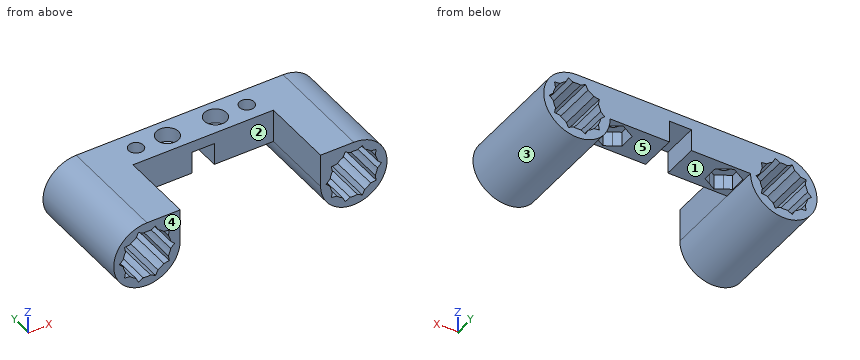
from build123d import *

# Parameters (mm, degrees)
F0_R            = 6.5
F1_DEPTH        = 25
F2_W            = 19
F2_H            = 9
F3_DEPTH        = 15
F4_R            = 2
F5_DEPTH        = 18.001
F7_DEPTH        = 25.001
F7_COPIES_COUNT = 10
F9_DEPTH        = 4
F10_DEPTH       = 5
F12_D           = 6
F12_DEPTH       = 4
F12_TIP         = 1.8025818571
F13_W           = 3
F13_H           = 6
F14_DEPTH       = 30.001


# Not quite as in the source:
# - a pattern or mirror of a feature is missing from the dataset's text; its kind, count and spacing are read off the source's solid


with BuildPart() as f1:
    # F0 (on Front) → F1 (new body)
    with BuildSketch(Plane.XZ):
        with BuildLine():
            Line((-19, 0), (0, 0))
            Line((0, 0), (0, 9))
            Line((0, 9), (-28, 9))
            ThreePointArc((-28, 9), (-21.6360389693, 6.3639610307), (-19, 0))
        make_face()
        with BuildLine():
            ThreePointArc((-28, 9), (-34.3639610307, -6.3639610307), (-19, 0))
            ThreePointArc((-19, 0), (-21.6360389693, 6.3639610307), (-28, 9))
        make_face()
        with Locations((-28, 0)):
            Circle(F0_R, mode=Mode.SUBTRACT)
    extrude(amount=F1_DEPTH)

    # F2 (on face) → F3 (cut)
    with BuildSketch(Plane.XZ.offset(25)):
        with Locations((-9.5, 4.5)):
            Rectangle(F2_W, F2_H)
    extrude(amount=-F3_DEPTH, mode=Mode.SUBTRACT)

    # F4 (on face) → F5 (cut, through all)
    with BuildSketch(Plane.XY.offset(9)):
        with Locations((-15, -5)):
            Circle(F4_R)
    extrude(amount=-F5_DEPTH, mode=Mode.SUBTRACT)

    # F6 (on face) → F7 (cut, through all)
    with BuildSketch(Plane.XZ.offset(25)):
        with BuildLine():
            Line((-21.5833333333, -1.0374916332), (-20.5, 0))
            Line((-20.5, 0), (-21.5833333333, 1.0374916332))
            ThreePointArc((-21.5833333333, 1.0374916332), (-21.5, 0), (-21.5833333333, -1.0374916332))
        make_face()
    f7 = extrude(amount=-F7_DEPTH, mode=Mode.SUBTRACT)

    # F7_copies: F7 ×10 about axis
    f7_copies_axis = Axis((-28, 0, 0), (0, 1, 0))
    for i in range(1, F7_COPIES_COUNT):
        add(f7.rotate(f7_copies_axis, i * 360 / F7_COPIES_COUNT), mode=Mode.SUBTRACT)

    # F8 (on face) → F9 (cut)
    with BuildSketch(Plane(origin=(0, 0, 0), x_dir=(1, 0, 0), z_dir=(0, 0, -1))):
        with BuildLine():
            ThreePointArc((-13.1250001976, 1.7524046217), (-11.7524047929, 3.1249999012), (-11.25, 5))
            ThreePointArc((-11.25, 5), (-11.7524048104, 6.8750001292), (-13.1250002583, 8.2475954133))
            ThreePointArc((-13.1250002583, 8.2475954133), (-15.0000000004, 8.75), (-16.8749997424, 8.2475954129))
            ThreePointArc((-16.8749997424, 8.2475954129), (-18.2475951898, 6.8750001288), (-18.75, 5))
            ThreePointArc((-18.75, 5), (-18.2475951898, 3.1249998712), (-16.8749997424, 1.7524045871))
            ThreePointArc((-16.8749997424, 1.7524045871), (-14.9999999654, 1.25), (-13.1250001976, 1.7524046217))
        make_face()
        with BuildLine():
            Line((-11.25, 2.8349364905), (-11.25, 5))
            ThreePointArc((-11.25, 5), (-11.7524047929, 3.1249999012), (-13.1250001976, 1.7524046217))
            Line((-13.1250001976, 1.7524046217), (-11.25, 2.8349364905))
        make_face()
        with BuildLine():
            ThreePointArc((-13.1250002583, 8.2475954133), (-11.7524048104, 6.8750001292), (-11.25, 5))
            Line((-11.25, 5), (-11.25, 7.1650635095))
            Line((-11.25, 7.1650635095), (-13.1250002583, 8.2475954133))
        make_face()
        with BuildLine():
            ThreePointArc((-16.8749997424, 8.2475954129), (-15.0000000004, 8.75), (-13.1250002583, 8.2475954133))
            Line((-13.1250002583, 8.2475954133), (-15, 9.3301270189))
            Line((-15, 9.3301270189), (-16.8749997424, 8.2475954129))
        make_face()
        with BuildLine():
            Line((-15, 0.6698729811), (-13.1250001976, 1.7524046217))
            ThreePointArc((-13.1250001976, 1.7524046217), (-14.9999999654, 1.25), (-16.8749997424, 1.7524045871))
            Line((-16.8749997424, 1.7524045871), (-15, 0.6698729811))
        make_face()
        with BuildLine():
            ThreePointArc((-18.75, 5), (-18.2475951898, 6.8750001288), (-16.8749997424, 8.2475954129))
            Line((-16.8749997424, 8.2475954129), (-18.75, 7.1650635095))
            Line((-18.75, 7.1650635095), (-18.75, 5))
        make_face()
        with BuildLine():
            Line((-18.75, 2.8349364905), (-16.8749997424, 1.7524045871))
            ThreePointArc((-16.8749997424, 1.7524045871), (-18.2475951898, 3.1249998712), (-18.75, 5))
            Line((-18.75, 5), (-18.75, 2.8349364905))
        make_face()
    extrude(amount=-F9_DEPTH, mode=Mode.SUBTRACT)

    # F10 (add): a face of the model
    f10_faces = [f1.faces().sort_by_distance(p)[0] for p in [
        (-34.1839610307, -25, -6.1839610307),
    ]]
    extrude(f10_faces, amount=F10_DEPTH)

    # F12
    with Locations(Plane.XY.offset(9)):
        with Locations((-6.5, -5)):
            Hole(F12_D / 2, depth=F12_DEPTH)
            with Locations((0, 0, -(F12_DEPTH + F12_TIP / 2))):  # 118° drill point
                Cone(0, F12_D / 2, F12_TIP, mode=Mode.SUBTRACT)

    # F13 (on face) → F14 (cut, through all)
    with BuildSketch(Plane(origin=(0, 0, 0), x_dir=(-1, 0, 0), z_dir=(0, 1, 0))):
        with Locations((1.5, 3)):
            Rectangle(F13_W, F13_H)
    extrude(amount=-F14_DEPTH, mode=Mode.SUBTRACT)

    # F15: F1 across plane


with BuildPart() as f1_1:
    add(f1.part)
    add(f1.part.mirror(Plane.YZ))


solid = f1_1.part
Verification items for the finished model (mm, model axes). Face numbers are marked on the shaded views. A direction names the side the tool comes from. Give positions to 0.01 mm unless a question says otherwise; leave off trailing zeros. Write each loop counter-clockwise with the first axis right and the second up, starting at its lowest first coordinate (ties: lowest second). Pieces come first, ordered by that corner, then holes. Notation, with made-up numbers: M -29.5,62 L 24.5,62 A23 ccw 24.5,80 Z; hole C 89,67 d8. An arc over 180 degrees is marked long. Put each result on its own line as item: value. Start each with the question number.
1. Go/stop test with flat-tipped pins: pin 1 Ø2 at (x, y) = (-21, -11.5) entering from -Z; pin 2 Ø3 at (y, z) = (-20.5, -4.5) entering from +X; pin 3 Ø5 at (x, z) = (-1.5, 2.5) entering from -Y; pin 4 Ø6 at (x, z) = (-26.5, -0.5) entering from +Y. Record where each tip stops, or that it passes through.
2. Scan lines: line 1 along X through (y, z) = (-26, -1.75); line 2 along Y through (x, z) = (6.5, 8.1); line 3 along X through (y, z) = (-14, -5.75). Record each from-to range of solid material in increasing order. Write a range as [from, to].
3. Draft check along X on the marked faces 4 and 5. Enter one of: +X half, -X half, draft (parallel to the pull), parting line (faces both ways), or undercut.
4. Set-up check for the marked faces 1, 2 and 3: record each of +Z, -Z, +X, -X, +Y, -Y from which the full face is reachable in a straight line by a thin tool's end or side.
5. Section check A-A (z = 2.25). Give the number of separate pieces and of enclosed holes in the cut face, and give its area (3 significant figures).
6. Section check B-B (x = -18). Record the cut outline in (y, z), and give its area (3 significant figures).
Answer list:
1. pin 1: z = -6.71
1. pin 2: x = 36.49
1. pin 3: y = -10
1. pin 4: through
2. line 1: [-36.83, -34.26], [-21.74, -19.17], [19.17, 21.74], [34.26, 36.83]
2. line 2: [-10, -8], [-2, 0]
2. line 3: [-34.92, -31.03], [-24.97, -21.08], [21.08, 24.97], [31.03, 34.92]
3. face 4: draft
3. face 5: undercut
4. face 1: -Z, +Y, -Y
4. face 2: +Z, -Z, -Y
4. face 3: +Y, -Y
5. separate pieces: 4
5. enclosed holes: 2
5. area: 554 mm2
6. outline: M -10,0 L -7.6,0 L -7.6,4 L -2.4,4 L -2.4,0 L 0,0 L 0,9 L -10,9 Z
6. area: 69.2 mm2
